Design review of the part built by this model. Coordinates are the model's own, in mm. A direction names the side the tool comes from. Give positions to 0.01 mm unless a question says otherwise; leave off trailing zeros. Loops run counter-clockwise (first coordinate to the right, second up) from the corner with the lowest first, then second, coordinate; pieces in that order, holes last. Notation, with made-up numbers: M 13,8 L 68,8 A22 cw 68,21 Z; hole C 37,-22.75 d10. An arc over 180 degrees is marked long. Use a Markdown table: item, result. Add a question column.
(1) Add section A-A, the plane z = 32.5. Give the boundary of the cut face in (x, y).
(2) For faces 5 (the face through (11.866, 0, 22)), 6 (the face through (6.866, 0, 22)), 7 (the face through (22.1, -7.3, 2)), 8 (the face through (9, -15, 22)), list the 3-axis set-ups (+Z, -Z, +X, -X, +Y, -Y) from which the entire face can be reached by the end or side of a thin tool; tool diameter is ignored.
(3) Add section D-D, the plane y = -7. Give the boundary of the cut face in (x, z).
(4) Draft analysis for pull direction Y (two halves, no side actions). For faces 1 (the face through (0, 0, 7)), 2 (the face through (9.331, -6.324, 31.763)), 3 (the face through (-2.994, -22.804, 4.465)), 4 (the face through (9.331, 7.676, 10.763)), state which applies: pulls with the +Y half, pulls with the -Y half, needs draft (parallel to the pull), parting line crosses it, or undercut.
(5) For probe 1 along Y at (x, z) = (10.15, 32.5); probe 2 along Y at (x, z) = (9, 11); probe 3 along X at (y, z) = (6, 32), list the stretches that pass through material, from the lowest coordinate up.
(6) Add section B-B, the plane y = 0. Give the boundary of the cut face in (x, z), then the cut area to 3 significant figures.
(7) Add section C-C, the plane x = 0. Give the boundary of the cut face in (y, z).
(8) Insertion check: pin 1 Ø1.6 at (y, z) = (-7, 32.5) entering from +X; pin 2 Ø5.5 at (x, z) = (10.5, 20.5) entering from -Y; pin 3 Ø9 at (y, z) = (-2.5, 26) entering from +X; pin 4 Ø3 at (y, z) = (-7, 11.5) entering from -X. Each pin has a flat end and moves straight along its axis. Give the tip position at first contact, or say it passes through.
Autodesk Inventor part; units mm, degrees
ref_plane "YZ Plane" through (0, 0, 0) normal (1, 0, 0) x (0, 1, 0)
ref_plane "XZ Plane" through (0, 0, 0) normal (0, 1, 0) x (-1, 0, 0)
ref_plane "XY Plane" through (0, 0, 0) normal (0, 0, 1) x (1, 0, 0)
sketch "Szkic1" plane through (0, 0, 0) normal (0, 0, 1) x (1, 0, 0)
  circle A0 centre (0, 0) radius 25
  dimension "d0" = 50
extrude "Wyciągnięcie proste1" add sketch "Szkic1" along normal blind 2
sketch "Szkic2" plane through (0, 0, 2) normal (0, 0, 1) x (1, 0, 0)
  circle A0 centre (0, 0) radius 23
  dimension "d3" = 46
extrude "Wyciągnięcie proste2" add sketch "Szkic2" along normal blind 5
sketch "Szkic3" plane through (0, 0, 7) normal (0, 0, 1) x (1, 0, 0)
  line L0 (6.8662, 15) -> (11.8662, 15)
  line L1 (11.8662, 15) -> (11.8662, -15)
  line L2 (11.8662, -15) -> (6.8662, -15)
  line L3 (6.8662, -15) -> (6.8662, 15)
  point P0 (0, 0)
  point P1 (6.8662, 0)
  dimension "d6" = 30
  dimension "d7" = 5
extrude "Wyciągnięcie proste3" add sketch "Szkic3" along normal blind 30
sketch "Szkic4" plane through (6.8662, -15, 7) normal (-1, 0, 0) x (0, 0, 1)
  circle A0 centre (4.5, 22) radius 1
  circle A1 centre (25.5, 22) radius 1
  circle A2 centre (4.5, 8) radius 1
  circle A3 centre (25.5, 8) radius 1
  line L0 (4.5, 22) -> (25.5, 22)
  line L1 (4.5, 22) -> (4.5, 8)
  line L2 (0, 30) -> (30, 30)
  line L3 (30, 30) -> (30, 0)
  point P0 (-7, 15)
  point P1 (15, 22)
  point P2 (15, 30)
  point P3 (4.5, 15)
  point P4 (30, 15)
  dimension "d10" = 2
  dimension "d11" = 2
  dimension "d12" = 2
  dimension "d13" = 2
  dimension "d14" = 14
  dimension "d15" = 21
extrude "Wyciągnięcie proste4" cut sketch "Szkic4" against normal blind 50
properties part number "camera_poprywka" material "Tworzywo sztuczne PET"
Established:
| question | item | result |
|---|---|---|
| 1 | outline | M 6.87,-15 L 11.87,-15 L 11.87,-8 L 6.87,-8 Z; M 6.87,-6 L 11.87,-6 L 11.87,6 L 6.87,6 Z; M 6.87,8 L 11.87,8 L 11.87,15 L 6.87,15 Z |
| 2 | face 5 | +Z, +X, +Y, -Y |
| 2 | face 6 | +Z, -X, +Y, -Y |
| 2 | face 7 | +Z |
| 2 | face 8 | +Z, +X, -X, -Y |
| 3 | outline | M -24,0 L 24,0 L 24,2 L 21.91,2 L 21.91,7 L 11.87,7 L 11.87,10.5 L 6.87,10.5 L 6.87,7 L -21.91,7 L -21.91,2 L -24,2 Z; M 6.87,12.5 L 11.87,12.5 L 11.87,31.5 L 6.87,31.5 Z; M 6.87,33.5 L 11.87,33.5 L 11.87,37 L 6.87,37 Z |
| 4 | face 1 | needs draft |
| 4 | face 2 | undercut |
| 4 | face 3 | parting line crosses it |
| 4 | face 4 | undercut |
| 5 | probe 1 | -15 to -8, -6 to 6, 8 to 15 |
| 5 | probe 2 | -15 to -7.87, -6.13 to 6.13, 7.87 to 15 |
| 5 | probe 3 | 6.87 to 11.87 |
| 6 | outline | M -25,0 L 25,0 L 25,2 L 23,2 L 23,7 L 11.87,7 L 11.87,37 L 6.87,37 L 6.87,7 L -23,7 L -23,2 L -25,2 Z |
| 6 | area | 480 mm^2 |
| 7 | outline | M -25,0 L 25,0 L 25,2 L 23,2 L 23,7 L -23,7 L -23,2 L -25,2 Z |
| 8 | pin 1 | through |
| 8 | pin 2 | y = -15 |
| 8 | pin 3 | x = 11.87 |
| 8 | pin 4 | x = 6.87 |
